Autodesk Fusion 360 part; units mm, degrees
sketch "Sketch1" plane through (0, 0, 0) normal (0, 1, 0) x (1, 0, 0)
  line L0 (0, 0) -> (215.9, 0)
  line L1 (215.9, 0) -> (215.9, 106.3625) construction
  line L2 (215.9, 106.3625) -> (0, 106.3625) construction
  line L3 (0, 106.3625) -> (0, 0)
  line L4 (23, 12) -> (193.9, 12) construction
  line L5 (193.9, 12) -> (193.9, 95.3625) construction
  line L6 (193.9, 95.3625) -> (23, 95.3625) construction
  line L7 (23, 95.3625) -> (23, 12) construction
  circle A0 centre (23, 95.3625) radius 3
  circle A1 centre (23, 12) radius 3
  circle A2 centre (193.9, 12) radius 3
  circle A3 centre (193.9, 95.3625) radius 3
  line L8 (431.8, 0) -> (431.8, 106.3625)
  line L9 (215.9, 0) -> (431.8, 0)
  line L10 (431.8, 106.3625) -> (215.9, 106.3625) construction
  line L11 (215.9, 106.3625) -> (215.9, 0) construction
  line L12 (409.8, 12) -> (409.8, 95.3625) construction
  line L13 (409.8, 95.3625) -> (238.9, 95.3625) construction
  circle A4 centre (409.8, 95.3625) radius 3
  circle A5 centre (238.9, 95.3625) radius 3
  circle A6 centre (409.8, 12) radius 3
  line L14 (238.9, 95.3625) -> (238.9, 12) construction
  line L15 (238.9, 12) -> (409.8, 12) construction
  circle A7 centre (238.9, 12) radius 3
  line L16 (215.9, 106.3625) -> (215.9, 212.725) construction
  line L17 (0, 106.3625) -> (215.9, 106.3625) construction
  line L18 (215.9, 212.725) -> (0, 212.725)
  line L19 (0, 212.725) -> (0, 106.3625)
  line L20 (193.9, 118.3625) -> (193.9, 201.725) construction
  line L21 (193.9, 201.725) -> (23, 201.725) construction
  circle A8 centre (193.9, 201.725) radius 3
  circle A9 centre (23, 201.725) radius 3
  circle A10 centre (193.9, 118.3625) radius 3
  line L22 (23, 201.725) -> (23, 118.3625) construction
  line L23 (23, 118.3625) -> (193.9, 118.3625) construction
  circle A11 centre (23, 118.3625) radius 3
  line L24 (431.8, 106.3625) -> (431.8, 212.725)
  line L25 (215.9, 106.3625) -> (431.8, 106.3625) construction
  line L26 (431.8, 212.725) -> (215.9, 212.725)
  line L27 (215.9, 212.725) -> (215.9, 106.3625) construction
  line L28 (409.8, 118.3625) -> (409.8, 201.725) construction
  line L29 (409.8, 201.725) -> (238.9, 201.725) construction
  circle A12 centre (409.8, 201.725) radius 3
  circle A13 centre (238.9, 201.725) radius 3
  circle A14 centre (409.8, 118.3625) radius 3
  line L30 (238.9, 201.725) -> (238.9, 118.3625) construction
  line L31 (238.9, 118.3625) -> (409.8, 118.3625) construction
  circle A15 centre (238.9, 118.3625) radius 3
  line L32 (33, 190.725) -> (183.9, 190.725)
  line L33 (183.9, 190.725) -> (183.9, 16)
  line L34 (183.9, 16) -> (33, 16)
  line L35 (33, 16) -> (33, 190.725)
  line L36 (248.9, 190.725) -> (399.8, 190.725)
  line L37 (399.8, 190.725) -> (399.8, 16)
  line L38 (399.8, 16) -> (248.9, 16)
  line L39 (248.9, 16) -> (248.9, 190.725)
  point P0 (215.9, 0)
  point P1 (0, 106.3625)
  point P2 (215.9, 106.3625)
  dimension "d35" = 106.3625
  dimension "d36" = 215.9
  dimension "d37" = 23
  dimension "d38" = 11
  dimension "d39" = 12
  dimension "d40" = 22
  dimension "d41" = 6
  dimension "d42" = 6
  dimension "d43" = 6
  dimension "d44" = 6
  dimension "d47" = 215.9
  dimension "d48" = 106.3625
  dimension "d49" = 10
  dimension "d51" = 11
  dimension "d52" = 4
  dimension "d53" = 10
  dimension "d54" = 10
  dimension "d55" = 11
  dimension "d56" = 10
  dimension "d57" = 4
extrude "Extrude1" add sketch "Sketch1" along normal blind 2.4
sketch "export" plane through (0, 2.4, 0) normal (0, 1, 0) x (-1, 0, 0)
  circle A0 centre (-23, -12) radius 3
  circle A1 centre (-23, -118.3625) radius 3
  line L0 (-399.8, -16) -> (-248.9, -16)
  line L1 (-248.9, -16) -> (-248.9, -190.725)
  line L2 (-248.9, -190.725) -> (-399.8, -190.725)
  line L3 (-399.8, -190.725) -> (-399.8, -16)
  circle A2 centre (-193.9, -12) radius 3
  circle A3 centre (-409.8, -118.3625) radius 3
  circle A4 centre (-23, -95.3625) radius 3
  circle A5 centre (-238.9, -201.725) radius 3
  circle A6 centre (-409.8, -201.725) radius 3
  circle A7 centre (-238.9, -118.3625) radius 3
  circle A8 centre (-23, -201.725) radius 3
  circle A9 centre (-193.9, -118.3625) radius 3
  line L4 (-183.9, -16) -> (-33, -16)
  line L5 (-33, -16) -> (-33, -190.725)
  line L6 (-33, -190.725) -> (-183.9, -190.725)
  line L7 (-183.9, -190.725) -> (-183.9, -16)
  circle A10 centre (-193.9, -95.3625) radius 3
  circle A11 centre (-193.9, -201.725) radius 3
  circle A12 centre (-409.8, -95.3625) radius 3
  circle A13 centre (-238.9, -12) radius 3
  circle A14 centre (-409.8, -12) radius 3
  circle A15 centre (-238.9, -95.3625) radius 3
  line L8 (-431.8, -212.725) -> (0, -212.725)
  line L9 (0, -212.725) -> (0, 0)
  line L10 (0, 0) -> (-431.8, 0)
  line L11 (-431.8, 0) -> (-431.8, -212.725)
equation "d35 = 8.375 in / 2"
equation "d36 = 17 in / 2"
equation "d42 = d41"
equation "d43 = d41"
equation "d44 = d41"
equation "d51 = d38"
equation "d52 = d51 - 7 mm"
equation "d53 = d49"
equation "d54 = d53"
equation "d55 = d51"
equation "d56 = d54"
equation "d57 = d52"
Geometry check sheet. Reference: the model listing, model coordinates, mm. Coordinates: 2 decimals unless noted, no trailing zeros. Write each loop counter-clockwise with the first axis right and the second up, starting at its lowest first coordinate (ties: lowest second). Pieces come first, ordered by that corner, then holes. Notation, with made-up numbers: (55.25, 79.5) -> (65.25, 79.5) arc R23 cw to (65.25, 90.5) -> close; hole circle Ø2 at (53.5, 4.5). An arc over 180 degrees is marked (long way). One line per question, with ' | ' between items.
1. Cross-section at A-A on z = -20.5. Record the cut outline in (x, y), and give its area (3 significant figures).
Answers:
outline: (0, 0) -> (33, 0) -> (33, 2.4) -> (0, 2.4) -> close; (183.9, 0) -> (248.9, 0) -> (248.9, 2.4) -> (183.9, 2.4) -> close; (399.8, 0) -> (431.8, 0) -> (431.8, 2.4) -> (399.8, 2.4) -> close | area: 312 mm²
2. Thickness scan on probe 1 along X at (y, z) = (1.7, -160); probe 2 along X at (y, z) = (1.6, -12); probe 3 along Z at (x, y) = (392.5, 1) (3 decimals). Record the ranges inside material, lowest first. Write a range as from..to.
Answers:
probe 1: x = 0..33, 183.9..248.9, 399.8..431.8 | probe 2: x = 0..20, 26..190.9, 196.9..235.9, 241.9..406.8, 412.8..431.8 | probe 3: z = -212.725..-190.725, -16..0
3. Cross-section at C-C on y = 0.45. State how many separate pieces and enclosed holes the cut face has, and give its area (3 significant figures).
Answers:
separate pieces: 1 | enclosed holes: 18 | area: 38,700 mm²
4. Cross-section at B-B on x = 305. Record the cut outline in (y, z) (3 decimals), and give its area (3 significant figures).
Answers:
outline: (0, -212.725) -> (2.4, -212.725) -> (2.4, -190.725) -> (0, -190.725) -> close; (0, -16) -> (2.4, -16) -> (2.4, 0) -> (0, 0) -> close | area: 91.2 mm²
